```python
from build123d import *

# Parameters (mm, degrees)
SCHIZZO1_R                   = 2.65
ESTRUSIONE_ESTRUSIONE1_DEPTH = 2.15
SCHIZZO2_R                   = 2.55
ESTRUSIONE_ESTRUSIONE2_DEPTH = 0.35
ESTRUSIONE_ESTRUSIONE3_DEPTH = 4
SCHIZZO4_R                   = 2.5
ESTRUSIONE_ESTRUSIONE4_DEPTH = 4
RIPETIZIONECIRCOLARE1_COUNT  = 45
SCHIZZO5_R                   = 1
TAGLIO_ESTRUSIONE1_DEPTH     = 7.5
SMUSSO1_SIZE                 = 0.25
SCHIZZO6_R                   = 2.75
SCHIZZO6_R_2                 = 2.45
TAGLIO_ESTRUSIONE2_DEPTH     = 0.35


with BuildPart() as part:
    # Schizzo1 → Estrusione-Estrusione1 (new body)
    with BuildSketch(Plane(origin=(0, 0, 0), x_dir=(1, 0, 0), z_dir=(0, 1, 0))):
        Circle(SCHIZZO1_R)
    extrude(amount=ESTRUSIONE_ESTRUSIONE1_DEPTH)

    # Schizzo2 → Estrusione-Estrusione2 (add)
    with BuildSketch(Plane(origin=(0, 2.15, 0), x_dir=(1, 0, 0), z_dir=(0, 1, 0))):
        Circle(SCHIZZO2_R)
    extrude(amount=ESTRUSIONE_ESTRUSIONE2_DEPTH)

    # Schizzo3 → Estrusione-Estrusione3 (add)
    with BuildSketch(Plane(origin=(0, 2.5, 0), x_dir=(1, 0, 0), z_dir=(0, 1, 0))):
        with BuildLine():
            Line((0, 2.65), (-0.087486608, 2.49846875))
            ThreePointArc((-0.087486608, 2.49846875), (0, 2.5), (0.087486608, 2.49846875))
            Line((0.087486608, 2.49846875), (0, 2.65))
        make_face()
    estrusione_estrusione3 = extrude(amount=ESTRUSIONE_ESTRUSIONE3_DEPTH)

    # Schizzo4 → Estrusione-Estrusione4 (add)
    with BuildSketch(Plane(origin=(0, 2.5, 0), x_dir=(1, 0, 0), z_dir=(0, 1, 0))):
        Circle(SCHIZZO4_R)
    extrude(amount=ESTRUSIONE_ESTRUSIONE4_DEPTH)

    # RipetizioneCircolare1: Estrusione-Estrusione3 ×45 about axis
    ripetizionecircolare1_axis = Axis((0, 0, 0), (0, 1, 0))
    for i in range(1, RIPETIZIONECIRCOLARE1_COUNT):
        add(estrusione_estrusione3.rotate(ripetizionecircolare1_axis, i * 360 / RIPETIZIONECIRCOLARE1_COUNT))

    # Schizzo5 → Taglio-Estrusione1 (cut, through all)
    with BuildSketch(Plane(origin=(0, 6.5, 0), x_dir=(1, 0, 0), z_dir=(0, 1, 0))):
        Circle(SCHIZZO5_R)
    extrude(amount=-TAGLIO_ESTRUSIONE1_DEPTH, mode=Mode.SUBTRACT)

    # Smusso1
    smusso1_edges = [part.edges().sort_by_distance(p)[0] for p in [
        (-1, 6.5, 0),
    ]]
    chamfer(smusso1_edges, length=SMUSSO1_SIZE)

    # Schizzo6 → Taglio-Estrusione2 (cut)
    with BuildSketch(Plane(origin=(0, 2.15, 0), x_dir=(1, 0, 0), z_dir=(0, 1, 0))):
        Circle(SCHIZZO6_R)
        Circle(SCHIZZO6_R_2, mode=Mode.SUBTRACT)
    extrude(amount=TAGLIO_ESTRUSIONE2_DEPTH, mode=Mode.SUBTRACT)


solid = part.part
```
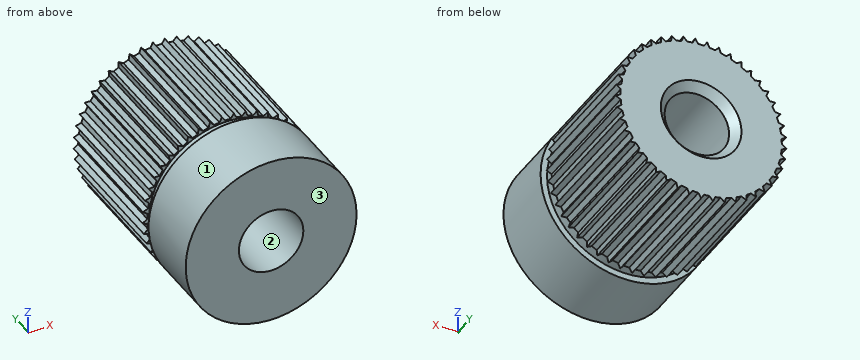
Build history of the part. All positions in model axes, mm. Face numbers are marked on the shaded views. Coordinates: 2 decimals unless noted, no trailing zeros. Order: outer loops, then holes, each group sorted by start corner. A loop starts at its lowest first (then second) coordinate and runs counter-clockwise, first axis right, second up.
Item 1: Mould opens along Z. For the marked faces 1, 2 and 3 say: released by +Z, released by -Z, zero draft, split by the parting line, or undercut.
Filled in:
face 1: split by the parting line
face 2: undercut
face 3: zero draft
Item 2: Drill centre lines: L1, parallel to Z at x = 0, y = 2; L2, parallel to X at y = 2.75, z = 2.2; L3, parallel to X at y = 1.5, z = -0.15. Where is each one in solid material? Low to high.
Filled in:
L1: z = -2.65 to -1, 1 to 2.65
L2: x = -1.25 to 1.25
L3: x = -2.65 to -0.99, 0.99 to 2.65
Item 3: Saw through at A-A on y = 1.25. List the corners of the cut face in (x, z), then the cut area to 3 significant figures.
Filled in:
outline: circle Ø5.3 at (0, 0); hole circle Ø2 at (0, 0)
area: 18.9 mm2
Item 4: Drop flat-ended pins along their axis: pin 1 Ø1.2 at (x, z) = (0, 0) entering from +Y; pin 2 Ø1.5 at (x, y) = (1.5, 5) entering from +Z. Give the stop position or say it passes through.
Filled in:
pin 1: passes through
pin 2: stops at z = 2.49
